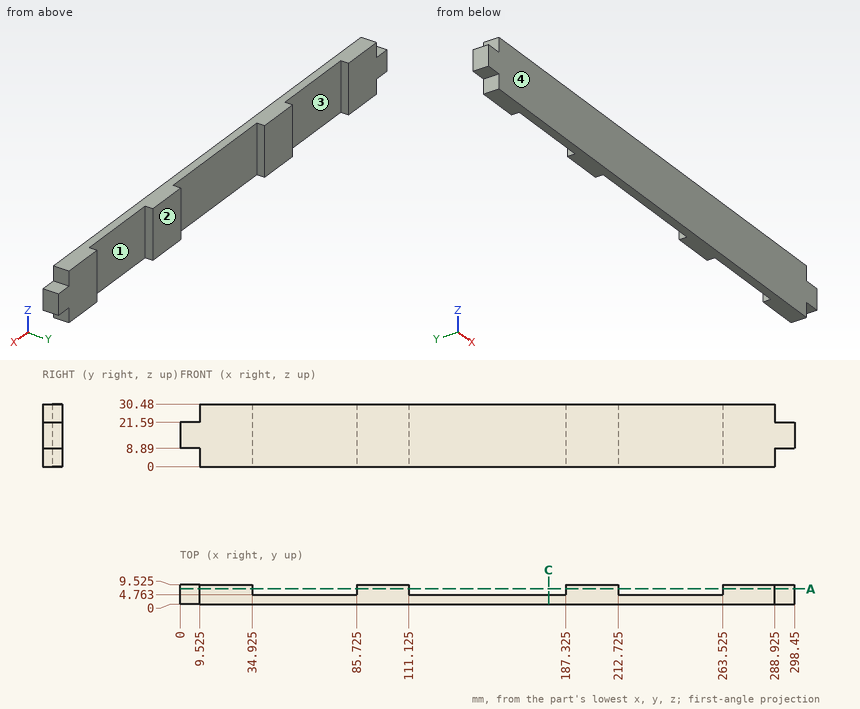
Part print with two shaded views. Sizes in mm from the minimum x, y, z corner. A direction names the side the tool comes from. Coordinates: 2 decimals unless noted, no trailing zeros. Write each loop counter-clockwise with the first axis right and the second up, starting at its lowest first coordinate (ties: lowest second). Pieces come first, ordered by that corner, then holes.
1. Drill centre lines: probe 1 along X at (y, z) = (8.25, 23) (1 decimal); probe 2 along Y at (x, z) = (176, 8.5); probe 3 along X at (y, z) = (1.5, 5.5) (1 decimal). Where is each one in solid material? Low to high.
Answer block:
probe 1: x = 9.5 to 34.9, 85.7 to 111.1, 187.3 to 212.7, 263.5 to 288.9
probe 2: y = 0 to 4.76
probe 3: x = 9.5 to 288.9
2. Pull direction X, two halves, no side cores. Call the marked faces 1 and 2: released by +X, released by -X, zero draft, split by the parting line, or undercut.
Answer block:
face 1: undercut
face 2: zero draft
3. Band-saw the part on A-A, the plane y = 7.5. Give the number of separate pieces and of enclosed holes in the cut face, and give its area (3 significant figures).
Answer block:
separate pieces: 4
enclosed holes: 0
area: 3,340 mm2
4. Drop flat-ended pins along their axis: pin 1 (3 mm diameter, centred on x = 5.5, y = 3.5, fed in from -Z); pin 2 (2.5 mm diameter, centred on y = 7.5, z = 8.5, fed in from +X); pin 3 (2.5 mm diameter, centred on y = 3.5, z = 3.5, fed in from +X) (1 decimal); pin 4 (9 mm diameter, centred on x = 72, z = 18.5, fed in from +Y). Give the stop position or say it passes through.
Answer block:
pin 1: stops at z = 8.89
pin 2: stops at x = 298.45
pin 3: stops at x = 288.9
pin 4: stops at y = 4.76
5. Band-saw the part on C-C, the plane x = 179. Give the cut face in (y, z).
Answer block:
outline: (0, 0) - (4.76, 0) - (4.76, 30.48) - (0, 30.48) - close
6. 3-axis set-ups, long thin cutter, end or side, ignore diameter. For the marked faces 3 and 4: which of +Z, -Z, +X, -X, +Y, -Y reach the whole face in a straight line?
Answer block:
face 3: +Z, -Z, +Y
face 4: +Z, -Z, +X, -X, -Y
